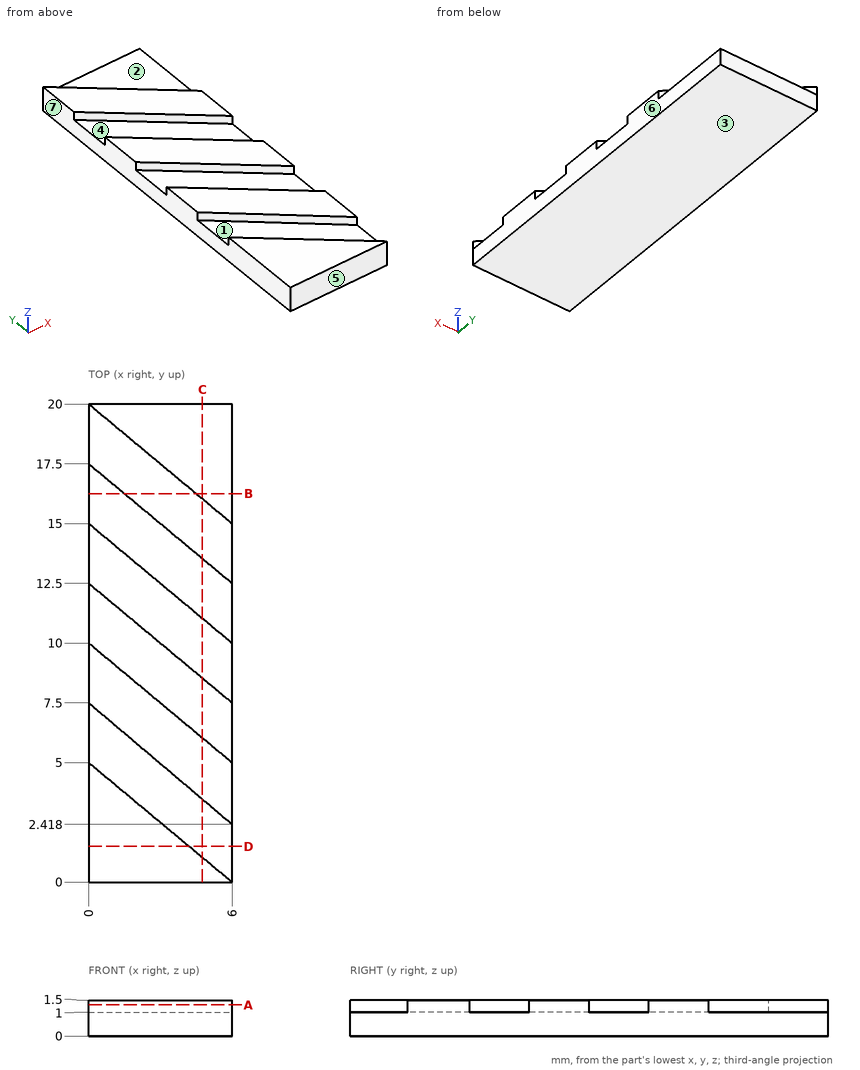
Answer from the drawing. Dimensions are ordinates in mm from the lowest x, y and z of the part. A direction names the side the tool comes from. Round coordinates to 2 decimals unless told otherwise and drop trailing zeros. Write each loop counter-clockwise with the first axis right and the second up, starting at its lowest first coordinate (ties: lowest second). Pieces come first, ordered by that corner, then holes. Notation, with made-up numbers: (16.25, 62) -> (74.25, 62) arc R12 cw to (74.25, 66) -> close; hole circle Ø7 at (62.5, 21.5). An arc over 180 degrees is marked (long way). Answer in a Markdown table with one row per item. Add a question column.
1) Consider line 1 (Y direction, x = 2, z = 1.35) (1 decimal); line 2 (Y direction, x = 0.75, z = 1.35) (1 decimal); line 3 (Z direction, x = 4.75, y = 11.25). Determine where each line is inside the solid, lowest interval first.
2) Find section D-D, the plane y = 1.5. Determine the outline of the cut face in (x, z).
3) Determine the mould class of the marked faces 4, 5, 6 and 7 for opening direction X: pulls with the +X half, pulls with the -X half, needs draft (parallel to the pull), parting line crosses it, or undercut.
4) Find section B-B, the plane y = 16.25. Determine the outline of the cut face in (x, z).
5) Find section C-C, the plane x = 4.75. Determine the outline of the cut face in (y, z).
6) Which of the six approach directions +Z, -Z, +X, -X, +Y, -Y give full straight-line access (tool end or side, diameter ignored) to the marked faces 1, 2 and 3?
7) Find section A-A, the plane z = 1.3. Determine the outline of the cut face in (x, y).
Findings below:
| question | item | result |
|---|---|---|
| 1 | line 1 | 0 to 3.3, 5.8 to 8.3, 10.8 to 13.3, 15.8 to 18.3 |
| 1 | line 2 | 0 to 4.4, 6.9 to 9.4, 11.9 to 14.4, 16.9 to 19.4 |
| 1 | line 3 | 0 to 1 |
| 2 | outline | (0, 0) -> (6, 0) -> (6, 1) -> (4.2, 1) -> (4.2, 1.5) -> (0, 1.5) -> close |
| 3 | face 4 | undercut |
| 3 | face 5 | needs draft |
| 3 | face 6 | pulls with the +X half |
| 3 | face 7 | pulls with the -X half |
| 4 | outline | (0, 0) -> (6, 0) -> (6, 1) -> (4.5, 1) -> (4.5, 1.5) -> (1.5, 1.5) -> (1.5, 1) -> (0, 1) -> close |
| 5 | outline | (0, 0) -> (20, 0) -> (20, 1) -> (16.04, 1) -> (16.04, 1.5) -> (13.54, 1.5) -> (13.54, 1) -> (11.04, 1) -> (11.04, 1.5) -> (8.54, 1.5) -> (8.54, 1) -> (6.04, 1) -> (6.04, 1.5) -> (3.48, 1.5) -> (3.48, 1) -> (1.04, 1) -> (1.04, 1.5) -> (0, 1.5) -> close |
| 6 | face 1 | +Z |
| 6 | face 2 | +Z, +X, +Y |
| 6 | face 3 | -Z, +X, -X, +Y, -Y |
| 7 | outline | (0, 0) -> (6, 0) -> (0, 5) -> close; (0, 7.5) -> (6, 2.42) -> (6, 5) -> (0, 10) -> close; (0, 12.5) -> (6, 7.5) -> (6, 10) -> (0, 15) -> close; (0, 17.5) -> (6, 12.5) -> (6, 15) -> (0, 20) -> close |
